Job drawing, mm, ordinate dimensions from the low corner. One solid piece. Coordinates: 2 decimals unless noted, no trailing zeros. Order: outer loops, then holes, each group sorted by start corner. A loop starts at its lowest first (then second) coordinate and runs counter-clockwise, first axis right, second up. Notation, with made-up numbers: (18, -3.5) - (64, -3.5) arc R28 cw to (64, 33.5) - close; hole circle Ø6 at (22, -25). An arc over 180 degrees is marked (long way). Use one line per item in the form item = value.
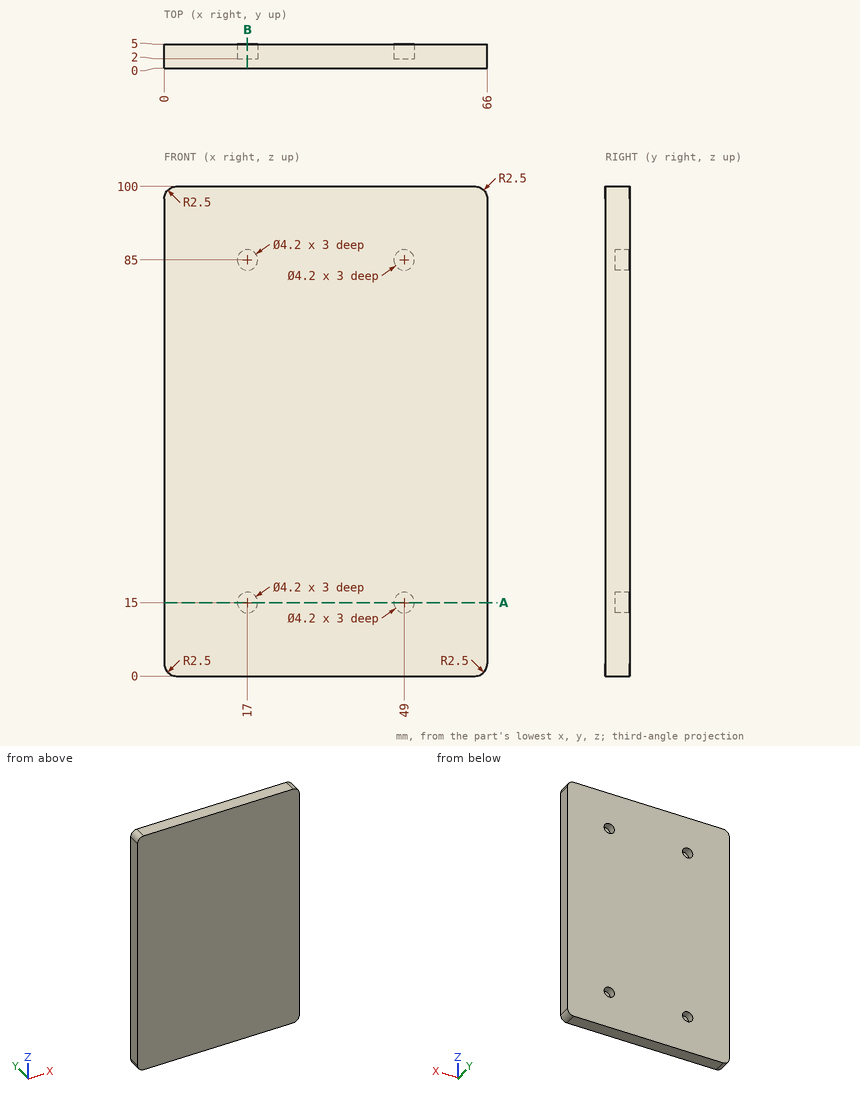
Item 1: Drop a flat-ended pin along its axis: pin 1 (1.3 mm diameter, centred on x = 49, z = 16, fed in from +Y). Give the stop position or say it passes through.
Derived:
pin_1 = 2
Item 2: Drill centre lines: line 1 (Z direction, x = 49, y = 3.8); line 2 (X direction, y = 3.7, z = 15); line 3 (Z direction, x = 18, y = 3.9). Where is each one in solid material? Low to high. Write a range as [from, to].
Derived:
line_1 = [0, 12.9], [17.1, 82.9], [87.1, 100]
line_2 = [0, 14.9], [19.1, 46.9], [51.1, 66]
line_3 = [0, 13.15], [16.85, 83.15], [86.85, 100]
Item 3: Cut at A-A, the plane z = 15. Write the cut outline in (x, y).
Derived:
outline = (0, 0) - (66, 0) - (66, 5) - (51.1, 5) - (51.1, 2) - (46.9, 2) - (46.9, 5) - (19.1, 5) - (19.1, 2) - (14.9, 2) - (14.9, 5) - (0, 5) - close
Item 4: Cut at B-B, the plane x = 17. Write the cut outline in (y, z).
Derived:
outline = (0, 0) - (5, 0) - (5, 12.9) - (2, 12.9) - (2, 17.1) - (5, 17.1) - (5, 82.9) - (2, 82.9) - (2, 87.1) - (5, 87.1) - (5, 100) - (0, 100) - close
